Job drawing, mm, ordinate dimensions from the low corner. One solid piece. A direction names the side the tool comes from. Coordinates: 2 decimals unless noted, no trailing zeros. Order: outer loops, then holes, each group sorted by start corner. A loop starts at its lowest first (then second) coordinate and runs counter-clockwise, first axis right, second up. Notation, with made-up numbers: (34.5, -37) - (81.5, -37) arc R37 cw to (81.5, 0) - close; hole circle Ø11 at (-16.5, 47.25). An arc over 180 degrees is marked (long way). Return JSON: item names as keys, results as strings.
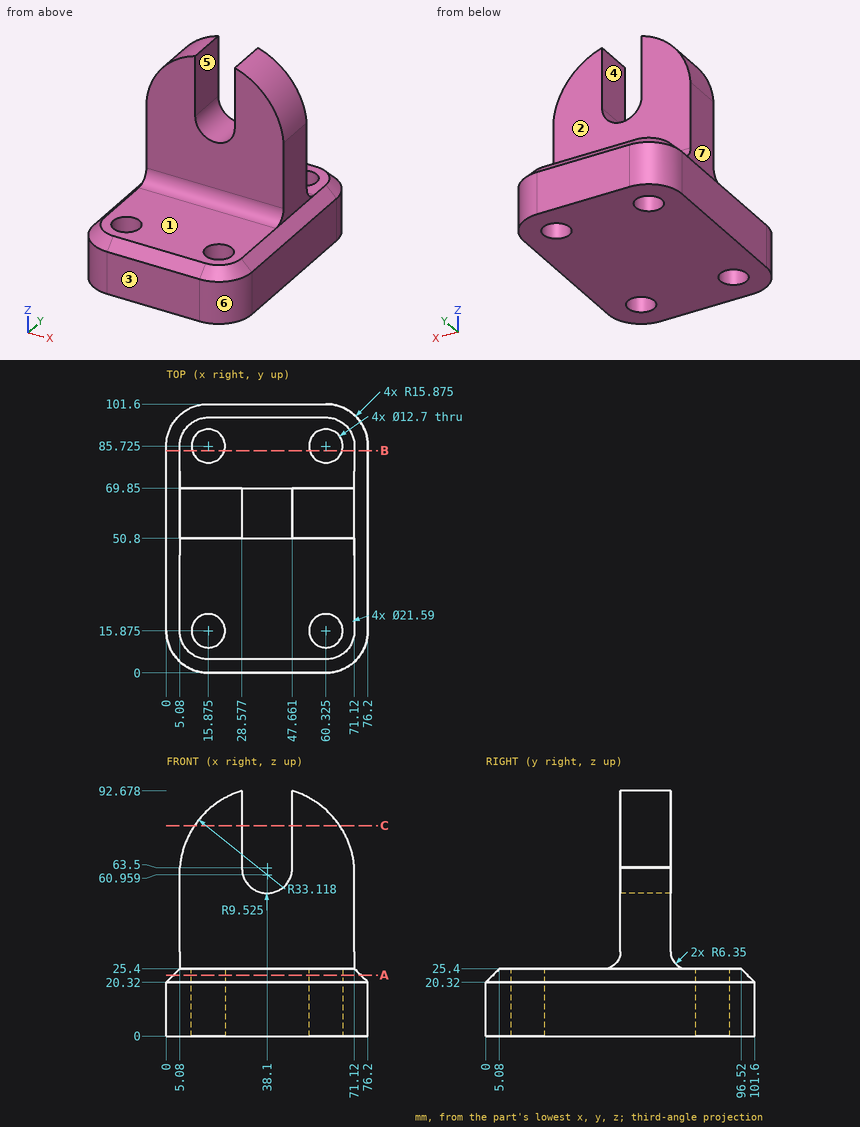
1. Mould opens along X. For the marked faces 4, 5, 6 and 7 say: pulls with the +X half, pulls with the -X half, needs draft (parallel to the pull), parting line crosses it, or undercut.
Check values:
{"face 4": "undercut", "face 5": "undercut", "face 6": "pulls with the +X half", "face 7": "pulls with the -X half"}
2. Cut at C-C on z = 79.5. Give the cut face in (x, y).
Check values:
{"outline": "(10.66, 50.8) - (28.58, 50.8) - (28.58, 69.85) - (10.66, 69.85) - close; (47.66, 50.8) - (65.54, 50.8) - (65.54, 69.85) - (47.66, 69.85) - close"}
3. Cut at A-A on z = 23. State how many separate pieces and enclosed holes the cut face has, plus the area to 3 significant figures.
Check values:
{"separate pieces": "1", "enclosed holes": "4", "area": "6,160 mm²"}
4. Drop flat-ended pins along their axis: pin 1 (5.5 mm diameter, centred on y = 62.5, z = 77.5, fed in from +X); pin 2 (16 mm diameter, centred on y = 65.5, z = 52.5, fed in from +X); pin 3 (18.5 mm diameter, centred on x = 45.5, z = 50, fed in from +Y); pin 4 (16.5 mm diameter, centred on x = 60.325, y = 15.875, fed in from -Z). Give the stop position or say it passes through.
Check values:
{"pin 1": "x = 68.21", "pin 2": "x = 71.12", "pin 3": "y = 69.85", "pin 4": "z = 0"}
5. Tool access for the marked faces 1, 2 and 3: list every direction of +Z, -Z, +X, -X, +Y, -Y with a clear straight run to the whole face (end or side of a thin tool).
Check values:
{"face 1": "+Z, +X, -X, -Y", "face 2": "+Z, +X, -X, +Y", "face 3": "+Z, -Z, +X, -X, -Y"}
6. Cut at B-B on y = 84. Give the cut face in (x, z), plus the area to 3 significant figures.
Check values:
{"outline": "(0, 0) - (9.76, 0) - (9.76, 25.4) - (5.08, 25.4) - (0, 20.32) - close; (21.99, 0) - (54.21, 0) - (54.21, 25.4) - (21.99, 25.4) - close; (66.44, 0) - (76.2, 0) - (76.2, 20.32) - (71.12, 25.4) - (66.44, 25.4) - close", "area": "1,290 mm²"}
7. Probe L1, parallel to Y at x = 16.5, z = 4 (1 decimal); L2, parallel to Y at x = 55.5, z = 18 (1 decimal); L3, parallel to X at y = 14, z = 13.5. List the from-to ranges inside material, lowest first.
Check values:
{"L1": "0 to 9.6, 22.2 to 79.4, 92 to 101.6", "L2": "0 to 11.7, 20 to 81.6, 89.9 to 101.6", "L3": "0.11 to 9.81, 21.94 to 54.26, 66.39 to 76.09"}
